from build123d import *

# Parameters (mm, degrees)
F3_R     = 2
F4_DEPTH = 12.6554723829


with BuildPart() as f1:
    # F0 (on Front) → F1 (revolve)
    with BuildSketch(Plane.XZ):
        Polygon((2.5, 0), (1.5, 0), (1.5, -5), (4.7805098866, -5), (6.7824029301, -5), (7, 0), align=None)
        Polygon((2.6259404258, 5.0502821417), (2.5, 0), (7, 0), (7, 5.0502821417), (4.8129702129, 5.0502821417), align=None)
        Polygon((2.7508953229, 10.0610440238), (2.6259404258, 5.0502821417), (4.8129702129, 5.0502821417), (7, 5.0502821417), (7, 10), align=None)
        Polygon((4.7805098866, -5), (3.9981069565, -22.9782505862), (6, -22.9782505862), (6.7824029301, -5), align=None)
        Polygon((3.5, 40.1005642833), (2.7508953229, 10.0610440238), (7, 10), (8.5, 40.1005642833), align=None)
    revolve(axis=Axis((0, 0, 25.1005642833), (0, 0, 1)))

    # F3 (on line) → F4 (join)
    with BuildSketch(Plane.YZ.offset(17.3129702129)):
        with Locations((0, 5.0502821417)):
            Circle(F3_R)
    extrude(amount=-F4_DEPTH)


solid = f1.part
Verification items for the finished model (mm, model axes). A direction names the side the tool comes from. Give positions to 0.01 mm unless a question says otherwise; leave off trailing zeros. Order: outer loops, then holes, each group sorted by start corner. A loop starts at its lowest first (then second) coordinate and runs counter-clockwise, first axis right, second up. Notation, with made-up numbers: M -11,47.5 L 25,47.5 A28 cw 25,76.5 Z; hole C 38.25,-4.5 d6. An arc over 180 degrees is marked long. Use one line per item in the form item = value. Start each with the question number.
Q1. Section check A-A (z = -14.5). Enter the section's corners in (x, y), then the cut area to 3 significant figures.
Q2. Mould release check, pull along Z, two halves, no side actions. Record for faces 4 (the cylindrical face through (-1.5, 0.07, -2.54)), 5 (the flat face through (1.42, -3.92, -22.978)), 6 (the flat face through (2, 0, 0)), 7 (the flat face through (-2, 0, -5)): +Z half, -Z half, draft (parallel to the pull), parting line (faces both ways), or undercut.
Q3. Scan lines: line 1 along X through (y, z) = (0.25, 27); line 2 along X through (y, z) = (3.5, -5.5); line 3 along Y through (x, z) = (0, -1.6). Record each from-to range of solid material in increasing order. Write a range as [from, to].
Q4. Access from +Z, -Z, +X, -X, +Y, -Y to the whole of each face (thin tool, end or side, straight path). Record for faces 1 (the flat face through (17.313, 0, 5)), 2 (the cylindrical face through (12.08, 1.91, 5.65)), 3 (the conical face through (4.18, 1.32, -14.11)).
Q5. Section check B-B (z = 25.5). Enter the section's corners in (x, y), then the cut area to 3 significant figures.
Q6. Go/stop test with flat-tipped pins: pin 1 Ø3 at (y, z) = (-1, 21) entering from -X; pin 2 Ø1 at (y, z) = (-5, -16.5) entering from +X; pin 3 Ø5 at (x, y) = (-2.5, 2) entering from -Z; pin 4 Ø2 at (y, z) = (-6, 15.5) entering from +X. Record where each tip stops, or that it passes through.
Evaluation:
q1.outline = C 0,0 d12.74; hole C 0,0 d8.73
q1.area = 67.5 mm2
q2.face_4 = draft
q2.face_5 = -Z half
q2.face_6 = +Z half
q2.face_7 = undercut
q3.line_1 = [-7.84, -3.16], [3.16, 7.84]
q3.line_2 = [-5.78, -3.22], [3.22, 5.78]
q3.line_3 = [-6.93, -1.5], [1.5, 6.93]
q4.face_1 = +Z, -Z, +X, +Y, -Y
q4.face_2 = +X
q4.face_3 = none
q5.outline = C 0,0 d15.54; hole C 0,0 d6.27
q5.area = 159 mm2
q6.pin_1 = -7.61
q6.pin_2 = 4.38
q6.pin_3 = -22.98
q6.pin_4 = 5.29
